Autodesk Inventor part; units mm, degrees
ref_plane "YZ Plane" through (0, 0, 0) normal (1, 0, 0) x (0, 1, 0)
ref_plane "XZ Plane" through (0, 0, 0) normal (0, 1, 0) x (-1, 0, 0)
ref_plane "XY Plane" through (0, 0, 0) normal (0, 0, 1) x (1, 0, 0)
sketch "Sketch1" plane through (0, 0, 0) normal (0, 0, 1) x (1, 0, 0)
  circle A0 centre (0, 0) radius 3.75
  line L0 (1.25, -6.25) -> (-1.25, -6.25)
  line L1 (-1.25, -6.25) -> (-1.25, 6.25) construction
  line L2 (-1.25, 6.25) -> (1.25, 6.25)
  line L3 (1.25, 6.25) -> (1.25, -6.25) construction
  circle A1 centre (0, 0) radius 5.25
  line L4 (1.25, -5.099) -> (1.25, -6.25)
  line L5 (-1.25, -6.25) -> (-1.25, -5.099)
  line L6 (-1.25, 6.25) -> (-1.25, 5.099)
  line L7 (1.25, 6.25) -> (1.25, 5.099)
  arc A2 (-1.25, -5.099) -> (1.25, -5.099) centre (0, 0) ccw
  arc A3 (1.25, 5.099) -> (-1.25, 5.099) centre (0, 0) ccw
  point P0 (0, 6.25)
  point P1 (1.25, 0)
  dimension "d1" = 7.5
  dimension "d10" = 2.5
  dimension "d11" = 12.5
  dimension "d12" = 10.5
extrude "Extrusion1" add sketch "Sketch1" along normal blind 10
sketch "Sketch5" plane through (0, 0, 0) normal (0, 0, -1) x (-1, 0, 0)
  circle A0 centre (0, 0) radius 3.75
  circle A1 centre (0, 0) radius 3.75
  line L0 (-1.25, -6.25) -> (-1.25, -5.099)
  line L1 (1.25, -6.25) -> (-1.25, -6.25)
  line L2 (1.25, -5.099) -> (1.25, -6.25)
  arc A2 (1.25, -5.099) -> (1.25, 5.099) centre (0, 0) ccw
  line L3 (1.25, 6.25) -> (1.25, 5.099)
  line L4 (-1.25, 6.25) -> (1.25, 6.25)
  line L5 (-1.25, 5.099) -> (-1.25, 6.25)
  arc A3 (-1.25, 5.099) -> (-1.25, -5.099) centre (0, 0) ccw
  circle A4 centre (0, 0) radius 1.5
  dimension "d13" = 3
extrude "Extrusion4" add sketch "Sketch5" along normal blind 2 contours A0 | L0 A3 L5 L4 L3 A2 L2 L1
sketch "Sketch6" plane through (0, 0, 0) normal (0, 0, 1) x (1, 0, 0)
  line L0 (0.625, 6.25) -> (-0.625, 6.25)
  line L1 (-0.625, 6.25) -> (-0.625, -6.25) construction
  line L2 (-0.625, -6.25) -> (0.625, -6.25)
  line L3 (0.625, -6.25) -> (0.625, 6.25) construction
  line L4 (-1.25, 6.25) -> (1.25, 6.25)
  circle A0 centre (0, 0) radius 1.5 construction
  arc A1 (0.625, 1.3636) -> (-0.625, 1.3636) centre (0, 0) ccw
  arc A2 (-0.625, -1.3636) -> (0.625, -1.3636) centre (0, 0) ccw
  line L5 (0.625, 6.25) -> (0.625, 1.3636)
  line L6 (-0.625, 6.25) -> (-0.625, 1.3636)
  line L7 (0.625, -1.3636) -> (0.625, -6.25)
  line L8 (-0.625, -1.3636) -> (-0.625, -6.25)
  point P0 (0, 0)
  point P1 (0, 6.25)
  point P2 (0.625, 0)
  dimension "d16" = 1.25
extrude "Extrusion5" add sketch "Sketch6" along normal blind 2
sketch "Sketch8" plane through (0, 0, -2) normal (0, 0, -1) x (-1, 0, 0)
  circle A0 centre (0, 0) radius 1.5
  line L0 (-1.25, -5.099) -> (-1.25, -6.25)
  line L1 (-1.25, -6.25) -> (1.25, -6.25)
  line L2 (1.25, -6.25) -> (1.25, -5.099)
  arc A1 (1.25, -5.099) -> (1.25, 5.099) centre (0, 0) ccw
  line L3 (1.25, 5.099) -> (1.25, 6.25)
  line L4 (1.25, 6.25) -> (-1.25, 6.25)
  line L5 (-1.25, 6.25) -> (-1.25, 5.099)
  arc A2 (-1.25, 5.099) -> (-1.25, -5.099) centre (0, 0) ccw
  circle A3 centre (0, 0) radius 3
  point P0 (0, 0)
  dimension "d22" = 6
extrude "Extrusion6" add sketch "Sketch8" along normal blind 4 contours A2 L5 L4 L3 A1 L2 L1 L0
properties part number "AA042" material "ABS Plastic"
Geometry check sheet. Reference: the model listing, model coordinates, mm. A direction names the side the tool comes from. Round coordinates to 2 decimals unless told otherwise and drop trailing zeros. Write each loop counter-clockwise with the first axis right and the second up, starting at its lowest first coordinate (ties: lowest second). Pieces come first, ordered by that corner, then holes.
Item 1: Access from +Z, -Z, +X, -X, +Y, -Y to the whole of each face (thin tool, end or side, straight path). Record for faces 1 (the face through (-1.25, -6, 2)), 2 (the face through (0, 1.5, 1)), 3 (the face through (1.25, -6, 2)), 4 (the face through (-0.625, -3, 1)), 5 (the face through (1.25, 6, 2)).
Determined:
face 1: +Z, -Z, -X, -Y
face 2: +Z, -Z
face 3: +Z, -Z, +X, -Y
face 4: +Z
face 5: +Z, -Z, +X, +Y
Item 2: Mould release check, pull along X, two halves, no side actions. Record for faces 6 (the face through (5.25, 0.1, 4.93)), 7 (the face through (0, -3, 2)), 8 (the face through (0, 6.25, 2)): +X half, -X half, draft (parallel to the pull), parting line (faces both ways), or undercut.
Determined:
face 6: +X half
face 7: undercut
face 8: draft
Item 3: Section check C-C (x = 0). Record the boundary of the cut face in (y, z), plus the area to 3 significant figures.
Determined:
outline: (-6.25, -6) - (-3, -6) - (-3, -2) - (-1.5, -2) - (-1.5, 2) - (-3.75, 2) - (-3.75, 10) - (-6.25, 10) - close; (1.5, -2) - (3, -2) - (3, -6) - (6.25, -6) - (6.25, 10) - (3.75, 10) - (3.75, 2) - (1.5, 2) - close
area: 104 mm2
Item 4: Go/stop test with flat-tipped pins: pin 1 Ø2 at (y, z) = (2.5, 1.5) entering from -X; pin 2 Ø1 at (y, z) = (-3, 1) entering from -X; pin 3 Ø0.9 at (x, y) = (-3, 1) entering from +Z. Record where each tip stops, or that it passes through.
Determined:
pin 1: stops at x = -5.03
pin 2: stops at x = -4.62
pin 3: stops at z = 0
Item 5: Material ranges on line 1 along Y through (x, z) = (0, -5.15); line 2 along X through (y, z) = (0, -1.55); line 3 along Y through (x, z) = (0, 2.5), recorded low to high.
Determined:
line 1: y = -6.25 to -3, 3 to 6.25
line 2: x = -5.25 to -1.5, 1.5 to 5.25
line 3: y = -6.25 to -3.75, 3.75 to 6.25
Item 6: Section check A-A (z = 6.75). Record the boundary of the cut face in (x, y), plus the area to 3 significant figures.
Determined:
outline: (-1.25, -6.25) - (1.25, -6.25) - (1.25, -5.1) arc R5.25 ccw to (1.25, 5.1) - (1.25, 6.25) - (-1.25, 6.25) - (-1.25, 5.1) arc R5.25 ccw to (-1.25, -5.1) - close; hole circle Ø7.5 at (0, 0)
area: 47.7 mm2
Item 7: Section check B-B (y = 0). Record the boundary of the cut face in (x, z).
Determined:
outline: (-5.25, -6) - (-3, -6) - (-3, -2) - (-1.5, -2) - (-1.5, 0) - (-3.75, 0) - (-3.75, 10) - (-5.25, 10) - close; (1.5, -2) - (3, -2) - (3, -6) - (5.25, -6) - (5.25, 10) - (3.75, 10) - (3.75, 0) - (1.5, 0) - close
Item 8: Section check D-D (z = -3.25). Record the boundary of the cut face in (x, y).
Determined:
outline: (-1.25, -6.25) - (1.25, -6.25) - (1.25, -5.1) arc R5.25 ccw to (1.25, 5.1) - (1.25, 6.25) - (-1.25, 6.25) - (-1.25, 5.1) arc R5.25 ccw to (-1.25, -5.1) - close; hole circle Ø6 at (0, 0)
